Design review of the part built by this model. Coordinates are the model's own, in mm. Coordinates: 2 decimals unless noted, no trailing zeros. Order: outer loops, then holes, each group sorted by start corner. A loop starts at its lowest first (then second) coordinate and runs counter-clockwise, first axis right, second up.
Autodesk Inventor part; units mm, degrees
ref_plane "YZ Plane" through (0, 0, 0) normal (1, 0, 0) x (0, 1, 0)
ref_plane "XZ Plane" through (0, 0, 0) normal (0, 1, 0) x (-1, 0, 0)
ref_plane "XY Plane" through (0, 0, 0) normal (0, 0, 1) x (1, 0, 0)
sketch "Sketch1" plane through (0, 0, 0) normal (0, 1, 0) x (-1, 0, 0)
  line L0 (0, 0) -> (50, 0)
  line L1 (50, 0) -> (50, -447.675)
  line L2 (50, -447.675) -> (0, -447.675)
  line L3 (0, -447.675) -> (0, 0)
  dimension "d0" = 50
  dimension "d1" = 447.675
extrude "Extrusion1" add sketch "Sketch1" along normal blind 4.7625
sketch "Sketch2" plane through (-50, 0, 0) normal (0, 0, 1) x (1, 0, 0)
  line L0 (1.1907, 3.5648) -> (1.1907, 1.1907)
  line L1 (50, 0) -> (0, 0)
  line L2 (50, 4.7625) -> (0, 4.7625)
  line L3 (1.1907, 1.1907) -> (48.8093, 1.1907)
  line L4 (1.1907, 3.5648) -> (48.8093, 3.5648)
  line L5 (48.8093, 3.5648) -> (48.8093, 1.1907)
  line L6 (50, 0) -> (50, 4.7625)
extrude "Extrusion2" add sketch "Sketch2" along normal blind 4.7625
sketch "Sketch3" plane through (0, 4.7625, 0) normal (0, 1, 0) x (1, 0, 0)
  line L0 (0, 0) -> (-25, 0)
  line L1 (-1.1907, 0) -> (-48.8093, 0)
  line L2 (-25, 65) -> (-19, 65)
  line L3 (-19, 65) -> (-25, 65)
  line L4 (-25, 65) -> (-31, 65)
  line L5 (-31, 65) -> (-31, 447.675)
  line L6 (0, 447.675) -> (-50, 447.675)
  line L7 (-19, 65) -> (-19, 447.675)
  line L8 (-19, 447.675) -> (-31, 447.675)
  dimension "d11" = 25
  dimension "d13" = 6
  dimension "d14" = 6
extrude "Extrusion3" cut sketch "Sketch3" against normal blind 10
sketch "Sketch4" plane through (-19, 4.7625, -65) normal (0, 0, -1) x (-1, 0, 0)
  line L0 (12, -4.7625) -> (0, -4.7625)
  line L1 (12, 0) -> (12, -4.7625)
  line L2 (0, 0) -> (12, 0)
  line L3 (0, 0) -> (0, -4.7625)
  point P0 (-19, -4.7625)
extrude "Extrusion4" add sketch "Sketch4" along normal blind 158.838
sketch "Sketch7" plane through (-19, 4.7625, -223.838) normal (0, 0, -1) x (-1, 0, 0)
  line L0 (0, -4.7625) -> (0, 0)
  line L1 (3.6185, 0) -> (3.6185, -4.7625)
  line L2 (3.6185, -4.7625) -> (8.3815, -4.7625)
  line L3 (8.3815, -4.7625) -> (8.3815, 0)
  line L4 (3.6185, 0) -> (8.3815, 0)
  line L5 (12, 0) -> (0, 0)
  line L6 (0, 0) -> (3.6185, 0)
  line L7 (0, -4.7625) -> (12, -4.7625)
  line L8 (3.6185, -4.7625) -> (0, -4.7625)
  line L9 (0, -4.7625) -> (0, 0)
  line L10 (8.3815, 0) -> (12, 0)
  line L11 (12, 0) -> (12, -4.7625)
  line L12 (12, 0) -> (12, -4.7625)
  line L13 (12, -4.7625) -> (8.3815, -4.7625)
  point P0 (-19, -4.7625)
  dimension "d20" = 4.763
extrude "Extrusion5" add sketch "Sketch7" along normal blind 223.837 contours L0 L5 L1 L7 | L3 L5 L11 L7
sketch "Sketch8" plane through (-50, 0, 0) normal (0, 0, 1) x (1, 0, 0)
  line L0 (26.187, 0) -> (26.187, 1.1907)
  line L1 (26.187, 1.1907) -> (23.813, 1.1907)
  line L2 (23.813, 1.1907) -> (23.813, 0)
  line L3 (26.187, 0) -> (23.813, 0)
  line L4 (23.813, 1.1907) -> (26.187, 1.1907)
  line L5 (1.1907, 1.1907) -> (1.1907, 3.5648)
  line L6 (1.1907, 2.3778) -> (48.8093, 2.3778)
  line L7 (48.8093, 1.1907) -> (1.1907, 1.1907)
  line L8 (26.187, 4.7555) -> (26.187, 3.5648)
  line L9 (26.187, 3.5648) -> (23.813, 3.5648)
  line L10 (23.813, 3.5648) -> (23.813, 4.7555)
  line L11 (26.187, 4.7555) -> (23.813, 4.7555)
  point P0 (0, 0)
  dimension "d25" = 2.374
extrude "Extrusion6" add sketch "Sketch8" along normal up to surface (4.7625 mm away)
sketch "Sketch9" plane through (0, 4.7625, 0) normal (0, 1, 0) x (1, 0, 0)
  line L0 (0, 0) -> (25, 0)
  line L1 (0, 447.675) -> (-22.6185, 447.675)
  line L2 (0, 447.675) -> (25, 447.675)
  line L3 (25, 447.675) -> (25, 0)
  line L4 (0, 0) -> (0, 447.675)
  line L5 (0, 0) -> (0, 447.675)
  line L6 (-50, 0) -> (0, 0)
  line L7 (-50, 0) -> (-75, 0)
  line L8 (-50, 447.675) -> (-75, 447.675)
  line L9 (-75, 447.675) -> (-75, 0)
  line L10 (-50, 0) -> (-50, 447.675)
  dimension "d28" = 25
extrude "Extrusion7" add sketch "Sketch9" against normal up to surface (4.7625 mm away)
sketch "Sketch10" plane through (0, 4.7625, 0) normal (0, 1, 0) x (1, 0, 0)
  line L0 (25, 0) -> (25, 447.675)
  line L1 (25, 0) -> (37.5, 0)
  line L2 (25, 447.675) -> (37.5, 447.675)
  line L3 (37.5, 447.675) -> (37.5, 0)
  line L4 (-75, 0) -> (25, 0)
  line L5 (25, 447.675) -> (-22.6185, 447.675)
  line L6 (25, 447.675) -> (25, 0)
  line L7 (-75, 0) -> (-75, 447.675)
  line L8 (-75, 0) -> (-87.5, 0)
  line L9 (-75, 447.675) -> (-87.5, 447.675)
  line L10 (-87.5, 447.675) -> (-87.5, 0)
  point P0 (0, 0)
  dimension "d31" = 12.5
extrude "Extrusion8" add sketch "Sketch10" against normal up to surface (4.7625 mm away)
sketch "Sketch11" plane through (-48.8093, 1.1907, 0) normal (0, 0, 1) x (1, 0, 0)
  line L0 (47.6185, 0) -> (24.9963, 0)
  line L1 (47.6185, 0) -> (85.1183, 0)
  line L2 (24.9963, 2.374) -> (47.6185, 2.374)
  line L3 (47.6185, 2.374) -> (85.1183, 2.374)
  line L4 (85.1183, 2.374) -> (85.1183, 0)
  line L5 (24.9963, -1.1907) -> (22.6223, -1.1907)
  line L6 (23.8093, -1.1907) -> (23.8093, 3.5648)
  line L7 (22.6223, 3.5648) -> (24.9963, 3.5648)
  line L8 (47.6185, 2.374) -> (47.6185, 0)
  line L9 (47.6185, 2.374) -> (47.6185, 0)
  line L10 (0, 0) -> (-37.4998, 0)
  line L11 (0, 2.374) -> (-37.4998, 2.374)
  line L12 (-37.4998, 2.374) -> (-37.4998, 0)
  line L13 (0, 2.374) -> (0, 0)
  point P0 (48.8093, -1.1907)
extrude "Extrusion9" add sketch "Sketch11" along normal up to surface (4.7625 mm away)
properties part number "Sustainable Chair_V1 - Leg" material "Foam Board - V3"
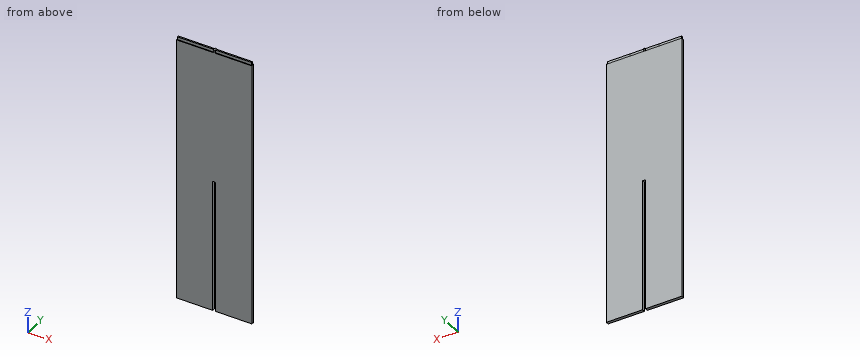
1. Add section B-B (y = 2.2). Give the boundary of the cut face in (x, z) (1 decimal).
2. Insertion check: pin 1 (4 mm diameter, centred on x = -36, z = 2.5, fed in from +Y); pin 2 (2.5 mm diameter, centred on x = -25.5, z = 3, fed in from +Y); pin 3 (1 mm diameter, centred on y = 4, z = 2.5, fed in from +X). Each pin has a flat end and moves straight along its axis. Give the tip position at first contact, or say it passes through.
3. To check wall thickness, follow line 1 (X direction, y = 0.4, z = -228); line 2 (Z direction, x = -18.5, y = 4) (3 decimals). State the ranges of each line that lie inside material, in increasing order.
4. Add section A-A (z = -373). Give the boundary of the cut face in (x, y).
Solution:
1. outline: (-87.5, -447.7) - (-27.4, -447.7) - (-27.4, -223.8) - (-22.6, -223.8) - (-22.6, -447.7) - (37.5, -447.7) - (37.5, 0) - (36.3, 0) - (36.3, 4.8) - (-86.3, 4.8) - (-86.3, 0) - (-87.5, 0) - close
2. pin 1: stops at y = 3.56
2. pin 2: stops at y = 4.76
2. pin 3: stops at x = 36.31
3. line 1: x = -87.5 to -27.38, -22.62 to 37.5
3. line 2: z = -447.675 to 0
4. outline: (-87.5, 0) - (-27.38, 0) - (-27.38, 4.76) - (-87.5, 4.76) - close; (-22.62, 0) - (37.5, 0) - (37.5, 4.76) - (-22.62, 4.76) - close
